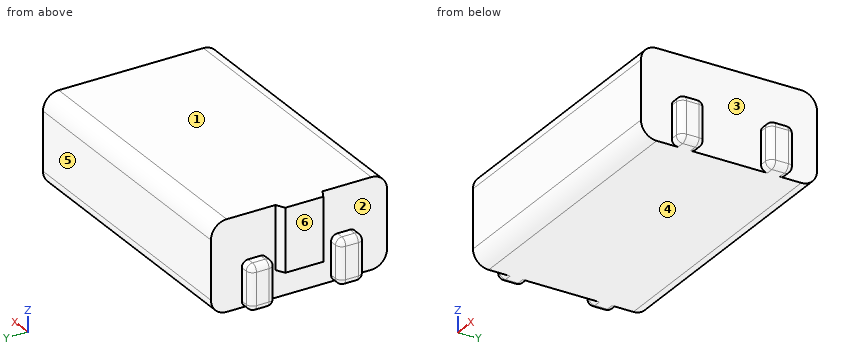
from build123d import *

# Parameters (mm, degrees)
F0_W     = 8.68
F0_H     = 5.6
F1_DEPTH = 2.85
F2_W     = 9.55
F2_H     = 0.8
F3_DEPTH = 1.425
F5_DEPTH = 2
F6_R     = 0.2
F7_R     = 0.5


with BuildPart() as f1:
    # F0 (on Top) → F1 (new body)
    with BuildSketch(Plane.XY):
        Rectangle(F0_W, F0_H)
    extrude(amount=F1_DEPTH)

    # F2 (on face) → F3 (join)
    with BuildSketch(Plane(origin=(0, 0, 0), x_dir=(1, 0, 0), z_dir=(0, 0, -1))):
        with Locations((0, 1.42)):
            Rectangle(F2_W, F2_H)
        with Locations((0, -1.42)):
            Rectangle(F2_W, F2_H)
    extrude(amount=-F3_DEPTH)

    # F4 (on face) → F5 (join)
    with BuildSketch(Plane.XY.offset(2.85)):
        Polygon((-4.34, -0.747284), (-4.34, 0), (-4.34, 0.747284), (-4.61323, 0.60448), (-4.61323, 0), (-4.61323, -0.60448), align=None)
    extrude(amount=-F5_DEPTH)

    # F6
    f6_edges = [f1.edges().sort_by_distance(p)[0] for p in [
        (-4.775, 1.82, 0.7125),
        (-4.775, 1.02, 0.7125),
        (-4.775, 1.42, 1.425),
        (-4.5575, 1.82, 1.425),
        (4.5575, 1.82, 1.425),
        (-4.5575, 1.02, 1.425),
        (4.5575, 1.02, 1.425),
        (-4.775, -1.02, 0.7125),
        (-4.775, -1.42, 1.425),
        (-4.775, -1.82, 0.7125),
        (-4.5575, -1.82, 1.425),
        (4.5575, -1.82, 1.425),
        (-4.5575, -1.02, 1.425),
        (4.5575, -1.02, 1.425),
        (-4.775, 1.42, 0),
        (4.5575, 1.02, 0),
        (-4.5575, 1.02, 0),
        (4.5575, 1.82, 0),
        (-4.5575, 1.82, 0),
        (4.5575, -1.02, 0),
        (-4.5575, -1.02, 0),
        (-4.775, -1.42, 0),
        (4.5575, -1.82, 0),
        (-4.5575, -1.82, 0),
        (4.775, -1.82, 0.7125),
        (4.775, -1.42, 1.425),
        (4.775, -1.02, 0.7125),
        (4.775, 1.02, 0.7125),
        (4.775, 1.42, 1.425),
        (4.775, 1.82, 0.7125),
        (4.775, -1.42, 0),
        (4.775, 1.42, 0),
    ]]
    fillet(f6_edges, radius=F6_R)

    # F7
    f7_edges = [f1.edges().sort_by_distance(p)[0] for p in [
        (0, -2.8, 2.85),
        (0, 2.8, 2.85),
        (0, 2.8, 0),
        (0, -2.8, 0),
    ]]
    fillet(f7_edges, radius=F7_R)


solid = f1.part
The listing builds one solid part. Answer for the finished solid, in the listing's coordinates (mm). Face numbers are marked on the shaded views. A direction names the side the tool comes from. Give positions to 0.01 mm unless a question says otherwise; leave off trailing zeros. Order: outer loops, then holes, each group sorted by start corner. A loop starts at its lowest first (then second) coordinate and runs counter-clockwise, first axis right, second up. Notation, with made-up numbers: (37, -35.5) - (71, -35.5) arc R29 cw to (71, -3.5) - close; hole circle Ø10 at (0.25, -35.75). An arc over 180 degrees is marked (long way). Use one line per item in the form item = value.
1) For the marked faces 1 and 2, determine the directions among +Z, -Z, +X, -X, +Y, -Y from which every point of the face is accessible in a straight line to the end or side of a thin tool.
Verdict:
face_1 = +Z, +X, -X, +Y, -Y
face_2 = -X
2) Each of these flat-tipped pins is pushed along its axis until it touches: pin 1 (0.9 mm diameter, centred on y = 1, z = 2, fed in from -X); pin 2 (1.5 mm diameter, centred on x = 2, z = 2.5, fed in from +Y). Where does it stop, or does it pass through?
Verdict:
pin_1 = -4.61
pin_2 = 2.8
3) Consider probe 1 along X at (y, z) = (2.5, 1.15); probe 2 along Y at (x, z) = (-2.5, 0.2); probe 3 along Z at (x, y) = (-1.75, -2.5). Determine where each line is inside the solid, lowest interval first. Write a range as [from, to].
Verdict:
probe_1 = [-4.34, 4.34]
probe_2 = [-2.7, 2.7]
probe_3 = [0.04, 2.81]
4) Find section A-A on y = 1.5. Determine the outline of the cut face in (x, z) (3 decimals).
Verdict:
outline = (-4.775, 0.2) arc R0.2 ccw to (-4.575, 0) - (4.575, 0) arc R0.2 ccw to (4.775, 0.2) - (4.775, 1.225) arc R0.2 ccw to (4.575, 1.425) - (4.34, 1.425) - (4.34, 2.85) - (-4.34, 2.85) - (-4.34, 1.425) - (-4.575, 1.425) arc R0.2 ccw to (-4.775, 1.225) - close
5) Find section C-C on y = 0.3. Determine the outline of the cut face in (x, z).
Verdict:
outline = (-4.61, 0.85) - (-4.34, 0.85) - (-4.34, 0) - (4.34, 0) - (4.34, 2.85) - (-4.61, 2.85) - close
6) The mould has two halves that part along Y. Classify the marked faces 3, 4, 5 and 6: released by +Y, released by -Y, zero draft, split by the parting line, or undercut.
Verdict:
face_3 = undercut
face_4 = zero draft
face_5 = released by +Y
face_6 = undercut
7) Find section B-B on z = 1.7. Determine the outline of the cut face in (x, y).
Verdict:
outline = (-4.61, -0.6) - (-4.34, -0.75) - (-4.34, -2.8) - (4.34, -2.8) - (4.34, 2.8) - (-4.34, 2.8) - (-4.34, 0.75) - (-4.61, 0.6) - close
8) Find section D-D on z = 2.5. Determine the outline of the cut face in (x, y), and give its area (3 significant figures).
Verdict:
outline = (-4.61, -0.6) - (-4.34, -0.75) - (-4.34, -2.78) - (4.34, -2.78) - (4.34, 2.78) - (-4.34, 2.78) - (-4.34, 0.75) - (-4.61, 0.6) - close
area = 48.6 mm^2
